Could you check a few things on this model? Use its own coordinates, in mm. A direction names the side the tool comes from. Round coordinates to 2 decimals unless told otherwise and drop trailing zeros. Loops run counter-clockwise (first coordinate to the right, second up) from the corner with the lowest first, then second, coordinate; pieces in that order, holes last.
Autodesk Inventor part; units mm, degrees
ref_plane "YZ Plane" through (0, 0, 0) normal (1, 0, 0) x (0, 1, 0)
ref_plane "XZ Plane" through (0, 0, 0) normal (0, 1, 0) x (-1, 0, 0)
ref_plane "XY Plane" through (0, 0, 0) normal (0, 0, 1) x (1, 0, 0)
sketch "Boceto1" plane through (0, 0, 0) normal (0, 0, 1) x (1, 0, 0)
  line L0 (0, 0) -> (195, 0)
  line L1 (195, 0) -> (195, -130)
  line L2 (195, -130) -> (0, -130)
  line L3 (-15, 0) -> (-15, -130)
  line L4 (0, -130) -> (-15, -130)
  line L5 (0, 0) -> (-15, 0)
  dimension "d1" = 130
extrude "Extrusión1" add sketch "Boceto1" along normal blind 5
sketch "Boceto2" plane through (0, 0, 5) normal (0, 0, 1) x (1, 0, 0)
  line L0 (-15, 0) -> (195, 0)
  line L1 (195, -130) -> (-15, -130)
  line L2 (30, 0) -> (40, 0)
  line L3 (100, 0) -> (110, 0)
  line L4 (170, 0) -> (180, 0)
  line L5 (170, -130) -> (180, -130)
  line L6 (100, -130) -> (110, -130)
  line L7 (30, -130) -> (40, -130)
  line L8 (40, 5) -> (40, 0)
  line L9 (40, -130) -> (40, -135)
  line L10 (30, -135) -> (30, -130)
  line L11 (30, 0) -> (30, 5)
  line L12 (110, 5) -> (110, 0)
  line L13 (110, -130) -> (110, -135)
  line L14 (100, -135) -> (100, -130)
  line L15 (100, 0) -> (100, 5)
  line L16 (180, 5) -> (180, 0)
  line L17 (180, -130) -> (180, -135)
  line L18 (170, -135) -> (170, -130)
  line L19 (170, 0) -> (170, 5)
  line L20 (30, 5) -> (30, 10)
  line L21 (40, 10) -> (40, 5)
  line L22 (100, 5) -> (100, 10)
  line L23 (110, 10) -> (110, 5)
  line L24 (170, 5) -> (170, 10)
  line L25 (180, 10) -> (180, 5)
  line L26 (40, -135) -> (40, -140)
  line L27 (30, -140) -> (30, -135)
  line L28 (110, -135) -> (110, -140)
  line L29 (100, -140) -> (100, -135)
  line L30 (180, -135) -> (180, -140)
  line L31 (170, -140) -> (170, -135)
  line L32 (170, 10) -> (180, 10)
  line L33 (30, 10) -> (40, 10)
  line L34 (100, 10) -> (110, 10)
  line L35 (180, -140) -> (170, -140)
  line L36 (110, -140) -> (100, -140)
  line L37 (40, -140) -> (30, -140)
extrude "Extrusión2" add sketch "Boceto2" against normal blind 5
sketch "Boceto3" plane through (0, 0, 5) normal (0, 0, 1) x (1, 0, 0)
  line L0 (195, 0) -> (195, -130)
  line L1 (180, 0) -> (195, 0)
  line L2 (-15, -130) -> (-15, 0)
  circle A0 centre (135, -120) radius 1.75
  circle A1 centre (160, -120) radius 1.75
  circle A2 centre (135, -10) radius 1.75
  circle A3 centre (160, -10) radius 1.75
  circle A4 centre (-4, -52.5) radius 1.75
  circle A5 centre (-4, -77.5) radius 1.75
  point P0 (30, 0)
  point P1 (30, -130)
  point P2 (0, 0)
  dimension "d20" = 3.5
  dimension "d21" = 3.5
  dimension "d22" = 3.5
  dimension "d23" = 3.5
  dimension "d24" = 3.5
  dimension "d25" = 3.5
  dimension "d26" = 25
  dimension "d27" = 25
  dimension "d28" = 25
  dimension "d29" = 10
  dimension "d30" = 10
  dimension "d31" = 150
  dimension "d32" = 150
  dimension "d33" = 52.5
  dimension "d34" = 199
extrude "Extrusión3" cut sketch "Boceto3" against normal blind 10
sketch "Boceto4" plane through (0, 0, 5) normal (0, 0, 1) x (1, 0, 0)
  line L0 (-1.6674, -130.3426) -> (-1.6674, -125.4313)
  line L1 (1.8326, -130.3426) -> (-1.6674, -130.3426)
  line L2 (1.8326, -125.4313) -> (1.8326, -130.3426)
  line L3 (-1.6674, -125.4313) -> (-2.6674, -125.4313)
  line L4 (-2.6674, -123.0313) -> (-1.6674, -123.0313)
  line L5 (-1.6674, -123.0313) -> (-1.6674, -120.2573)
  line L6 (1.8326, -120.2573) -> (1.8326, -123.0313)
  line L7 (2.8326, -125.4313) -> (1.8326, -125.4313)
  line L8 (2.8326, -123.0313) -> (2.8326, -125.4313)
  line L9 (1.8326, -123.0313) -> (2.8326, -123.0313)
  line L10 (1.8326, -120.2573) -> (-1.6674, -120.2573)
  line L11 (-2.6674, -125.4313) -> (-2.6674, -123.0313)
  line L12 (167.9972, -120.715) -> (164.4972, -120.715)
  line L13 (167.9972, -120.715) -> (167.9972, -123.4891)
  line L14 (164.4972, -123.4891) -> (164.4972, -120.715)
  line L15 (167.9972, -123.4891) -> (168.9972, -123.4891)
  line L16 (168.9972, -123.4891) -> (168.9972, -125.8891)
  line L17 (163.4972, -125.8891) -> (163.4972, -123.4891)
  line L18 (164.4972, -125.8891) -> (163.4972, -125.8891)
  line L19 (168.9972, -125.8891) -> (167.9972, -125.8891)
  line L20 (163.4972, -123.4891) -> (164.4972, -123.4891)
  line L21 (164.4972, -130.8004) -> (164.4972, -125.8891)
  line L22 (167.9972, -130.8004) -> (164.4972, -130.8004)
  line L23 (167.9972, -125.8891) -> (167.9972, -130.8004)
  line L24 (71.7006, -120.3125) -> (68.2006, -120.3125)
  line L25 (71.7006, -120.3125) -> (71.7006, -123.0866)
  line L26 (68.2006, -123.0866) -> (68.2006, -120.3125)
  line L27 (71.7006, -123.0866) -> (72.7006, -123.0866)
  line L28 (72.7006, -123.0866) -> (72.7006, -125.4866)
  line L29 (67.2006, -125.4866) -> (67.2006, -123.0866)
  line L30 (68.2006, -125.4866) -> (67.2006, -125.4866)
  line L31 (72.7006, -125.4866) -> (71.7006, -125.4866)
  line L32 (67.2006, -123.0866) -> (68.2006, -123.0866)
  line L33 (68.2006, -130.3979) -> (68.2006, -125.4866)
  line L34 (71.7006, -130.3979) -> (68.2006, -130.3979)
  line L35 (71.7006, -125.4866) -> (71.7006, -130.3979)
  line L36 (1.8326, -9.3206) -> (-1.6674, -9.3206)
  line L37 (1.8326, -9.3206) -> (1.8326, -6.5466)
  line L38 (-1.6674, -6.5466) -> (-1.6674, -9.3206)
  line L39 (1.8326, -6.5466) -> (2.8326, -6.5466)
  line L40 (2.8326, -6.5466) -> (2.8326, -4.1466)
  line L41 (-2.6674, -4.1466) -> (-2.6674, -6.5466)
  line L42 (-1.6674, -4.1466) -> (-2.6674, -4.1466)
  line L43 (2.8326, -4.1466) -> (1.8326, -4.1466)
  line L44 (-2.6674, -6.5466) -> (-1.6674, -6.5466)
  line L45 (-1.6674, 0.7647) -> (-1.6674, -4.1466)
  line L46 (1.8326, 0.7647) -> (-1.6674, 0.7647)
  line L47 (1.8326, -4.1466) -> (1.8326, 0.7647)
  line L48 (168.9375, -3.8347) -> (167.9375, -3.8347)
  line L49 (167.9375, -3.8347) -> (167.9375, 1.0766)
  line L50 (167.9375, 1.0766) -> (164.4375, 1.0766)
  line L51 (167.9375, -6.2347) -> (168.9375, -6.2347)
  line L52 (167.9375, -9.0087) -> (167.9375, -6.2347)
  line L53 (164.4375, 1.0766) -> (164.4375, -3.8347)
  line L54 (164.4375, -3.8347) -> (163.4375, -3.8347)
  line L55 (163.4375, -3.8347) -> (163.4375, -6.2347)
  line L56 (163.4375, -6.2347) -> (164.4375, -6.2347)
  line L57 (164.4375, -6.2347) -> (164.4375, -9.0087)
  line L58 (167.9375, -9.0087) -> (164.4375, -9.0087)
  line L59 (168.9375, -6.2347) -> (168.9375, -3.8347)
  line L60 (72.7006, -6.4914) -> (72.7006, -4.0914)
  line L61 (72.7006, -4.0914) -> (71.7006, -4.0914)
  line L62 (71.7006, -6.4914) -> (72.7006, -6.4914)
  line L63 (71.7006, -4.0914) -> (71.7006, 0.8199)
  line L64 (71.7006, -9.2654) -> (71.7006, -6.4914)
  line L65 (71.7006, 0.8199) -> (68.2006, 0.8199)
  line L66 (68.2006, 0.8199) -> (68.2006, -4.0914)
  line L67 (71.7006, -9.2654) -> (68.2006, -9.2654)
  line L68 (68.2006, -6.4914) -> (68.2006, -9.2654)
  line L69 (68.2006, -4.0914) -> (67.2006, -4.0914)
  line L70 (67.2006, -4.0914) -> (67.2006, -6.4914)
  line L71 (67.2006, -6.4914) -> (68.2006, -6.4914)
  line L72 (170, 10) -> (170, 0)
  point P0 (0, 0)
  dimension "d37" = 3.5
  dimension "d38" = 3.5
  dimension "d39" = 3.5
  dimension "d45" = 2.0625
extrude "Extrusión4" cut sketch "Boceto4" against normal blind 10
properties part number "pieza central base superior"
Item 1: We'd pull the mould along X, two halves only. Please class faces 1 (the flat face through (180, -135, 3)), 2 (the flat face through (138, -130, 2)), 3 (the flat face through (89, -64, 0)): released by +X, released by -X, zero draft, split by the parting line, or undercut.
Results list:
face 1: released by +X
face 2: undercut
face 3: zero draft
Item 2: If we section it at A-A, the plane z = 1.3: Count the separate pieces of the cut face and the enclosed holes in it, then the cut area to 3 significant figures.
Results list:
separate pieces: 1
enclosed holes: 6
area: 27,600 mm2
Item 3: If we section it at B-B, the plane x = 148: Please give me the cut outline in (y, z).
Results list:
outline: (-130, 0) - (0, 0) - (0, 5) - (-130, 5) - close
Item 4: If I drill on line 1 along Y through (x, z) = (-4, 2.6); line 2 along X through (y, z) = (-8, 0.7); line 3 along X through (y, z) = (-127, 2.85), over which ranges is the centre line in solid material (lowest first)?
Results list:
line 1: y = -130 to -79.25, -75.75 to -54.25, -50.75 to 0
line 2: x = -15 to -1.67, 1.83 to 68.2, 71.7 to 164.44, 167.94 to 195
line 3: x = -15 to -1.67, 1.83 to 68.2, 71.7 to 164.5, 168 to 195
Item 5: Will these pins go through, and if not, where does the flat tip stop? pin 1 (1 mm diameter, centred on x = 166, z = 2, fed in from -Y) (3 decimals); pin 2 (1.5 mm diameter, centred on x = 59, z = 2.5, fed in from +Y).
Results list:
pin 1: stops at y = -120.715
pin 2: stops at y = 0
Item 6: For faces 4 (the flat face through (68.201, -2, 3)), 5 (the flat face through (30, -135, 3)), 6 (the flat face through (110, -135, 3)), which set-ups out of +Z, -Z, +X, -X, +Y, -Y let a thin tool reach every point of the face, with its end or its side?
Results list:
face 4: +Z, -Z, +Y
face 5: +Z, -Z, -X, -Y
face 6: +Z, -Z, -Y
